from build123d import *

# Parameters (mm, degrees)
F0_R     = 1.5
F1_DEPTH = 26
F2_W     = 10
F2_H     = 1.5
F3_DEPTH = 26
F4_R     = 0.75
F5_DEPTH = 28.9


with BuildPart() as f1:
    # F0 (on Front) → F1 (new body)
    with BuildSketch(Plane.XZ):
        Circle(F0_R)
    extrude(amount=F1_DEPTH)

    # F2 (on Front) → F3 (join)
    with BuildSketch(Plane.XZ):
        with Locations((-5, -0.75)):
            Rectangle(F2_W, F2_H)
    extrude(amount=F3_DEPTH)

    # F4 (on Front) → F5 (cut)
    with BuildSketch(Plane.XZ):
        Circle(F4_R)
    extrude(amount=F5_DEPTH, mode=Mode.SUBTRACT)


solid = f1.part
The listing builds one solid part. Answer for the finished solid, in the listing's coordinates (mm). A direction names the side the tool comes from. Round coordinates to 2 decimals unless told otherwise and drop trailing zeros. Write each loop counter-clockwise with the first axis right and the second up, starting at its lowest first coordinate (ties: lowest second). Pieces come first, ordered by that corner, then holes. Notation, with made-up numbers: M 74,-20 L 106,-20 A21 ccw 106,12 Z; hole C 14.25,53 d11. An arc over 180 degrees is marked long. Write each question's results on one line, items separated by ' | '. Start each with the question number.
(1) The part is cut by section C-C, the plane x = -6.5. Write down the section's boundary in (y, z).
(2) This flat-tipped pin is pushed along its axis until it touches: P1, Ø3, axis at x = -6.5, y = -17.5, coming from the +Z side. Where does it stop, or does it pass through?
(3) Find the intervals of material crossed by line 1 (Z direction, x = 0, y = -7.5); line 2 (Z direction, x = -7.25, y = -21.25); line 3 (X direction, y = -15.25, z = 0.1), in increasing order.
(4) Determine the mould class of faces 1 (the cylindrical face through (-0.75, -12.82, 0.03)), 2 (the flat face through (-10, -13, -1)), 3 (the flat face through (-4, -26, -1)) for opening direction X: +X half, -X half, draft (parallel to the pull), parting line (faces both ways), or undercut.
(5) The part is cut by section B-B, the plane y = -20.5. Write down the section's boundary in (x, z), and give its area (3 significant figures).
(6) The part is cut by section A-A, the plane z = -0.5. Write down the section's boundary in (x, y), and give its area (3 significant figures).
(7) For faces 4 (the flat face through (-6, -13, 0)), 5 (the flat face through (-4, 0, -1)), determine the directions among +Z, -Z, +X, -X, +Y, -Y from which every point of the face is accessible in a straight line to the end or side of a thin tool.
Worked answers:
1) outline: M -26,-1.5 L 0,-1.5 L 0,0 L -26,0 Z
2) P1: stops at z = 0
3) line 1: z = -1.5 to -0.75, 0.75 to 1.5 | line 2: z = -1.5 to 0 | line 3: x = -1.5 to -0.74, 0.74 to 1.5
4) face 1: undercut | face 2: -X half | face 3: draft
5) outline: M -10,-1.5 L 0,-1.5 A1.5 ccw long -1.5,0 L -10,0 Z; hole C 0,0 d1.5 | area: 18.5 mm²
6) outline: M -10,-26 L -0.56,-26 L -0.56,0 L -10,0 Z; M 0.56,-26 L 1.41,-26 L 1.41,0 L 0.56,0 Z | area: 268 mm²
7) face 4: +Z, -X, +Y, -Y | face 5: +Z, -Z, +X, -X, +Y
